CAD build for the part. Positions are in the model's coordinates, mm. Coordinates: 2 decimals unless noted, no trailing zeros. Write each loop counter-clockwise with the first axis right and the second up, starting at its lowest first coordinate (ties: lowest second). Pieces come first, ordered by that corner, then holes. Notation, with made-up numbers: (-10.75, 59) - (41.25, 59) arc R36 ccw to (41.25, 95) - close; hole circle Ø6 at (74, -1). An arc over 180 degrees is marked (long way). One line per question, with ' | ' between items. Start each with the question number.
1. Band-saw the part on B-B, the plane y = 3.5. Write the cut outline in (x, z) (3 decimals).
2. Band-saw the part on C-C, the plane x = 255.5. Write the cut outline in (y, z) (3 decimals), then the cut area to 3 significant figures.
3. Probe line 1 (Y direction, x = 12.7, z = 10.5); line 2 (Z direction, x = 102.5, y = 19) (3 decimals); line 3 (Y direction, x = 252, z = -9) (3 decimals). List the from-to ranges inside material, lowest first.
4. Band-saw the part on D-D, the plane z = 5.75. Write the cut outline in (x, y) (3 decimals), then the cut area to 3 significant figures.
5. Band-saw the part on A-A, the plane x = 215.9. Give the number of separate pieces and of enclosed holes in the cut face, then the cut area to 3 significant figures.
from build123d import *

# Parameters (mm, degrees)
F0_W     = 50.8
F0_H     = 25.4
F0_W_2   = 44.45
F0_H_2   = 19.05
F1_DEPTH = 304.8
F3_D     = 5.1054
F5_D     = 5.1054


# Not quite as in the source:
# - a feature names something its author has since deleted; it is built from what else it names


with BuildPart() as f1:
    # F0 (on Right) → F1 (new body)
    with BuildSketch(Plane.YZ):
        Rectangle(F0_W, F0_H)
        Rectangle(F0_W_2, F0_H_2, mode=Mode.SUBTRACT)
    extrude(amount=F1_DEPTH)

    # F3 (through all)
    with Locations(Plane.XZ.offset(25.4)):
        with Locations((215.9, 0), (63.5, 0), (88.9, 0), (165.1, 0), (38.1, 0), (12.7, 0), (114.3, 0), (292.1, 0), (139.7, 0), (241.3, 0), (190.5, 0), (266.7, 0)):
            Hole(F3_D / 2)

    # F5 (through all)
    with Locations(Plane.XY.offset(12.7)):
        with Locations((114.3, 12.7), (38.1, -12.7), (63.5, 12.7), (38.1, 12.7), (88.9, -12.7), (266.7, -12.7), (215.9, 12.7), (139.7, -12.7), (63.5, -12.7), (190.5, 12.7), (241.3, -12.7), (114.3, -12.7), (12.7, 12.7), (292.1, 12.7), (12.7, -12.7), (190.5, -12.7), (88.9, 12.7), (241.3, 12.7), (165.1, -12.7), (165.1, 12.7), (139.7, 12.7), (266.7, 12.7), (292.1, -12.7), (215.9, -12.7)):
            Hole(F5_D / 2)


solid = f1.part
Filled in:
1) outline: (0, -12.7) - (304.8, -12.7) - (304.8, -9.525) - (0, -9.525) - close; (0, 9.525) - (304.8, 9.525) - (304.8, 12.7) - (0, 12.7) - close
2) outline: (-25.4, -12.7) - (25.4, -12.7) - (25.4, 12.7) - (-25.4, 12.7) - close; hole (-22.225, -9.525) - (22.225, -9.525) - (22.225, 9.525) - (-22.225, 9.525) - close | area: 444 mm²
3) line 1: y = -25.4 to -15.25, -10.15 to 10.15, 15.25 to 25.4 | line 2: z = -12.7 to -9.525, 9.525 to 12.7 | line 3: y = -25.4 to -22.225, 22.225 to 25.4
4) outline: (0, -25.4) - (304.8, -25.4) - (304.8, -22.225) - (0, -22.225) - close; (0, 22.225) - (304.8, 22.225) - (304.8, 25.4) - (0, 25.4) - close | area: 1,940 mm²
5) separate pieces: 6 | enclosed holes: 0 | area: 346 mm²
